Design review of the part shown in the three views and the two pictorial views. Dimensions are in mm from the part's minimum x, y and z. Give positions to 0.01 mm unless a question says otherwise; leave off trailing zeros. Write each loop counter-clockwise with the first axis right and the second up, starting at its lowest first coordinate (ties: lowest second). Pieces come first, ordered by that corner, then holes.
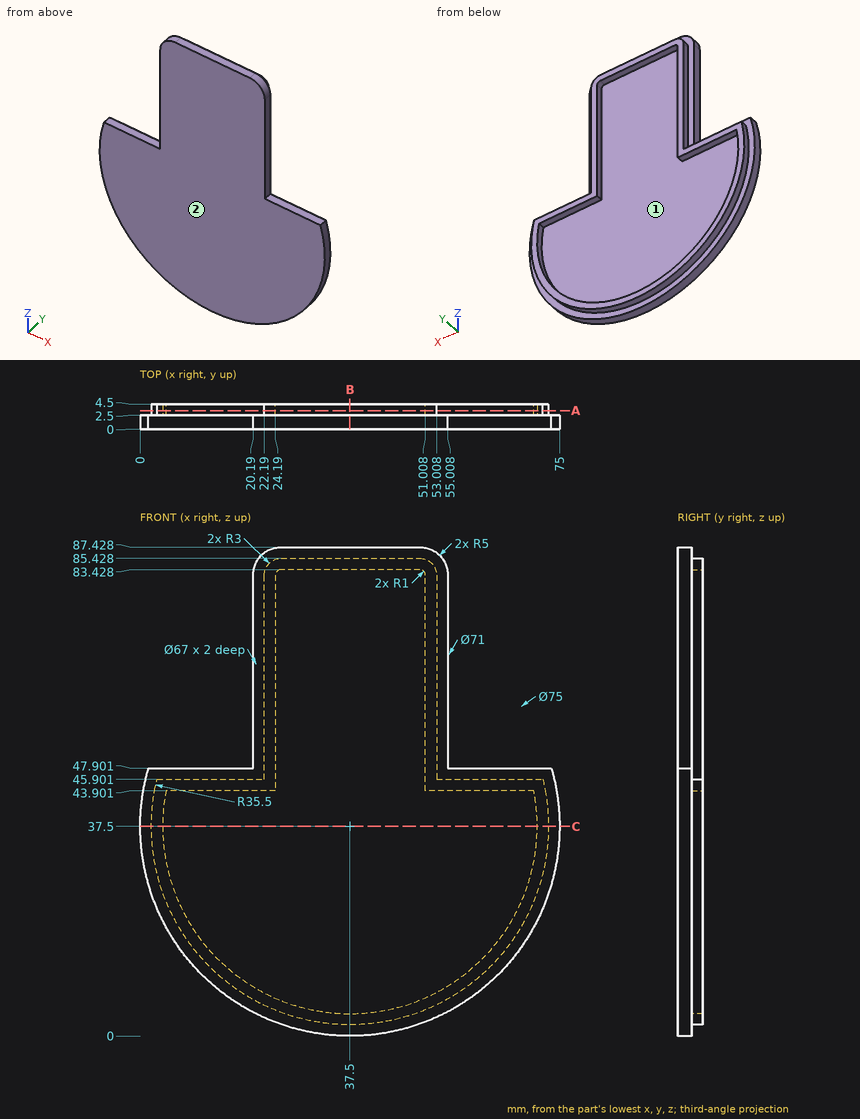
(1) Consider section C-C, the plane z = 37.5. Give the boundary of the cut face in (x, y).
Resolved:
outline: (0, 0) - (75, 0) - (75, 2.5) - (73, 2.5) - (73, 4.5) - (71, 4.5) - (71, 2.5) - (4, 2.5) - (4, 4.5) - (2, 4.5) - (2, 2.5) - (0, 2.5) - close
(2) Mouldability with a two-part tool opening along Z and no side actions: class the marked faces 1 and 2 as pulls with the +Z half, pulls with the -Z half, needs draft (parallel to the pull), parting line crosses it, or undercut.
Resolved:
face 1: undercut
face 2: needs draft
(3) Consider section B-B, the plane x = 37.5. Give the boundary of the cut face in (y, z).
Resolved:
outline: (0, 0) - (2.5, 0) - (2.5, 2) - (4.5, 2) - (4.5, 4) - (2.5, 4) - (2.5, 83.43) - (4.5, 83.43) - (4.5, 85.43) - (2.5, 85.43) - (2.5, 87.43) - (0, 87.43) - close
(4) Consider section A-A, the plane y = 3.3. Give the boundary of the cut face in (x, z), then the cut area to 3 significant figures.
Resolved:
outline: (3.01, 45.9) arc R35.5 ccw (long way) to (71.99, 45.9) - (53.01, 45.9) - (53.01, 82.43) arc R3 ccw to (50.01, 85.43) - (25.19, 85.43) arc R3 ccw to (22.19, 82.43) - (22.19, 45.9) - close; hole (4.62, 43.9) arc R33.5 ccw (long way) to (70.38, 43.9) - (51.01, 43.9) - (51.01, 82.43) arc R1 ccw to (50.01, 83.43) - (25.19, 83.43) arc R1 ccw to (24.19, 82.43) - (24.19, 43.9) - close
area: 536 mm2
(5) To check wall thickness, follow L1, parallel to X at y = 3, z = 37.5; L2, parallel to X at y = 3, z = 73; L3, parallel to Y at x = 33, z = 10.5. State the ranges of each line that lie inside material, in increasing order.
Resolved:
L1: x = 2 to 4, 71 to 73
L2: x = 22.19 to 24.19, 51.01 to 53.01
L3: y = 0 to 2.5
(6) Clearance check with flat-ended pins moving along their axes: P1, Ø1.6, axis at x = 31.5, y = 3.5, coming from the +Z side; P2, Ø1, axis at x = 65, y = 2.5, coming from the +Z side; P3, Ø3, axis at x = 37, z = 29.5, coming from the +Y side. State where each tip first meets the part, or that it passes through.
Resolved:
P1: stops at z = 85.43
P2: stops at z = 47.9
P3: stops at y = 2.5
